The model under review builds one solid part; all positions refer to its coordinate system, in mm. Face numbers are marked on the shaded views. A direction names the side the tool comes from. Round coordinates to 2 decimals unless told otherwise and drop trailing zeros. Loops run counter-clockwise (first coordinate to the right, second up) from the corner with the lowest first, then second, coordinate; pieces in that order, holes last. Notation, with made-up numbers: (64.25, -17) -> (103.25, -17) arc R27 cw to (103.25, 0) -> close; hole circle Ø10 at (0.5, 63). An arc over 180 degrees is marked (long way). Use a Markdown table: item, result. Add a question column.
1) Mouldability with a two-part tool opening along Y and no side actions: class the marked faces 1, 2, 3 and 4 as released by +Y, released by -Y, zero draft, split by the parting line, or undercut.
2) Wall thickness on probe 1 along Y at (x, z) = (38.5, 15.5); probe 2 along X at (y, z) = (134.5, 10); probe 3 along Y at (x, z) = (46.5, 10.75): over which ranges is each line inside the solid? List them lowest first.
3) Insertion check: pin 1 (2.5 mm diameter, centred on x = 51.5, y = 134, fed in from +Z); pin 2 (2.5 mm diameter, centred on x = 51, y = 74, fed in from +Z); pin 3 (3 mm diameter, centred on y = 99.5, z = 8.5, fed in from -X). Each pin has a flat end and moves straight along its axis. Give the tip position at first contact, or say it passes through.
4) Consider section D-D on y = 122.5. Give the boundary of the cut face in (x, z).
5) For the marked faces 5, 6 and 7, list the 3-axis set-ups (+Z, -Z, +X, -X, +Y, -Y) from which the entire face can be reached by the end or side of a thin tool; tool diameter is ignored.
6) Consider section B-B on z = 1.5. State how many separate pieces and enclosed holes the cut face has, plus the area to 3 significant figures.
7) Consider section A-A on z = 8. Give the boundary of the cut face in (x, y) (3 decimals), plus the area to 3 significant figures.
8) Consider section C-C on x = 70. Give the boundary of the cut face in (y, z).
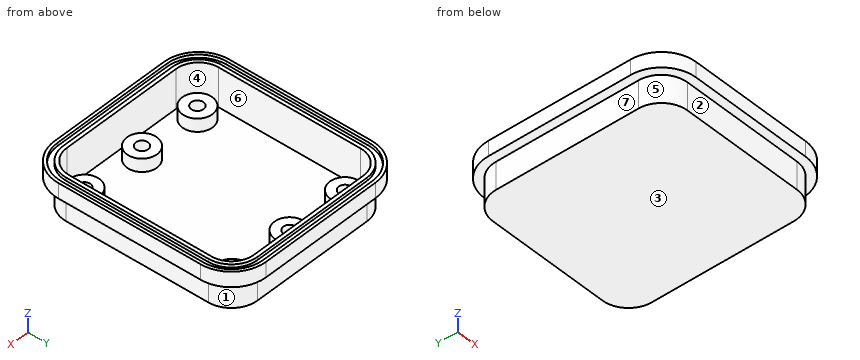
from build123d import *

# Parameters (mm, degrees)
BOSS_EXTRUDE1_DEPTH  = 16.51
SHELL1_T             = 1.524
SKETCH2_R            = 6.35
SKETCH2_R_2          = 2.608000118
BOSS_EXTRUDE2_DEPTH  = 5.5
BOSS_EXTRUDE9_DEPTH  = 1.3208
BOSS_EXTRUDE10_START = 5.08
BOSS_EXTRUDE10_DEPTH = 5.08


with BuildPart() as part:
    # Sketch1 → Boss-Extrude1 (new body)
    with BuildSketch(Plane.XY):
        with BuildLine():
            Line((26.034999985, 143.509994751), (78.104997498, 143.509994751))
            ThreePointArc((78.104997498, 143.509994751), (84.840189588, 140.720186842), (87.629997498, 133.984994751))
            Line((87.629997498, 133.984994751), (87.629997498, 73.787000793))
            ThreePointArc((87.629997498, 73.787000793), (84.840189588, 67.051808703), (78.104997498, 64.262000793))
            Line((78.104997498, 64.262000793), (26.034999985, 64.262000793))
            ThreePointArc((26.034999985, 64.262000793), (19.299807894, 67.051808703), (16.509999985, 73.787000793))
            Line((16.509999985, 73.787000793), (16.509999985, 133.984994751))
            ThreePointArc((16.509999985, 133.984994751), (19.299807894, 140.720186842), (26.034999985, 143.509994751))
        make_face()
    extrude(amount=BOSS_EXTRUDE1_DEPTH)

    # Shell1
    shell1_openings = [part.faces().sort_by_distance(p)[0] for p in [
        (52.069998741, 103.885997772, 16.51),
    ]]
    offset(amount=SHELL1_T, openings=shell1_openings, kind=Kind.INTERSECTION)

    # Sketch2 → Boss-Extrude2 (add)
    # profile 1 of 6: a face of its own
    with BuildSketch(Plane.XY):
        with Locations(Location((25.292, 135.128, 0), (0, 0, 180))):
            Circle(SKETCH2_R)
        with Locations((25.292, 135.128)):
            Circle(SKETCH2_R_2, mode=Mode.SUBTRACT)
    # profile 2 of 6: a face of its own
    with BuildSketch(Plane.XY):
        with Locations(Location((51.708, 135.128, 0), (0, 0, 180))):
            Circle(SKETCH2_R)
        with Locations((51.708, 135.128)):
            Circle(SKETCH2_R_2, mode=Mode.SUBTRACT)
    # profile 3 of 6: a face of its own
    with BuildSketch(Plane.XY):
        with Locations(Location((79.14, 135.128, 0), (0, 0, 180))):
            Circle(SKETCH2_R)
        with Locations((79.14, 135.128)):
            Circle(SKETCH2_R_2, mode=Mode.SUBTRACT)
    # profile 4 of 6: a face of its own
    with BuildSketch(Plane.XY):
        with Locations(Location((25.292, 72.644, 0), (0, 0, 180))):
            Circle(SKETCH2_R)
        with Locations((25.292, 72.644)):
            Circle(SKETCH2_R_2, mode=Mode.SUBTRACT)
    # profile 5 of 6: a face of its own
    with BuildSketch(Plane.XY):
        with Locations(Location((51.708, 72.644, 0), (0, 0, 180))):
            Circle(SKETCH2_R)
        with Locations((51.708, 72.644)):
            Circle(SKETCH2_R_2, mode=Mode.SUBTRACT)
    # profile 6 of 6: a face of its own
    with BuildSketch(Plane.XY):
        with Locations(Location((79.14, 72.644, 0), (0, 0, 180))):
            Circle(SKETCH2_R)
        with Locations((79.14, 72.644)):
            Circle(SKETCH2_R_2, mode=Mode.SUBTRACT)
    extrude(amount=BOSS_EXTRUDE2_DEPTH)



with BuildPart() as body_2:
    # Sketch7 → Boss-Extrude9 (new body)
    with BuildSketch(Plane.XY.offset(16.51)):
        with BuildLine():
            Line((92.786197498, 73.787000793), (92.786197498, 133.984994751))
            ThreePointArc((92.786197498, 133.984994751), (88.486173574, 144.366170827), (78.104997498, 148.666194751))
            Line((78.104997498, 148.666194751), (26.034999985, 148.666194751))
            ThreePointArc((26.034999985, 148.666194751), (15.653823909, 144.366170827), (11.353799985, 133.984994751))
            Line((11.353799985, 133.984994751), (11.353799985, 73.787000793))
            ThreePointArc((11.353799985, 73.787000793), (15.653823909, 63.405824718), (26.034999985, 59.105800793))
            Line((26.034999985, 59.105800793), (78.104997498, 59.105800793))
            ThreePointArc((78.104997498, 59.105800793), (88.486173574, 63.405824718), (92.786197498, 73.787000793))
        make_face()
        with BuildLine():
            ThreePointArc((26.034999985, 147.396194751), (16.551849521, 143.468145215), (12.623799985, 133.984994751))
            Line((12.623799985, 133.984994751), (12.623799985, 73.787000793))
            ThreePointArc((12.623799985, 73.787000793), (16.551849521, 64.30385033), (26.034999985, 60.375800793))
            Line((26.034999985, 60.375800793), (78.104997498, 60.375800793))
            ThreePointArc((78.104997498, 60.375800793), (87.588147961, 64.30385033), (91.516197498, 73.787000793))
            Line((91.516197498, 73.787000793), (91.516197498, 133.984994751))
            ThreePointArc((91.516197498, 133.984994751), (87.588147961, 143.468145215), (78.104997498, 147.396194751))
            Line((78.104997498, 147.396194751), (26.034999985, 147.396194751))
        make_face(mode=Mode.SUBTRACT)
    extrude(amount=-BOSS_EXTRUDE9_DEPTH)


with BuildPart() as part_1:
    add(part.part)

    add(body_2.part)  # Boss-Extrude10 merges body 2
    # Sketch8 → Boss-Extrude10 (add)
    # profile 1 of 2: a face of its own
    with BuildSketch(Plane(origin=(0, 0, 15.1892), x_dir=(-1, 0, 0), z_dir=(0, 0, -1)).offset(BOSS_EXTRUDE10_START)):
        with BuildLine():
            ThreePointArc((-78.104997498, 148.666194751), (-88.486173574, 144.366170827), (-92.786197498, 133.984994751))
            Line((-92.786197498, 133.984994751), (-92.786197498, 73.787000793))
            ThreePointArc((-92.786197498, 73.787000793), (-88.486173574, 63.405824718), (-78.104997498, 59.105800793))
            Line((-78.104997498, 59.105800793), (-26.034999985, 59.105800793))
            ThreePointArc((-26.034999985, 59.105800793), (-15.653823909, 63.405824718), (-11.353799985, 73.787000793))
            Line((-11.353799985, 73.787000793), (-11.353799985, 133.984994751))
            ThreePointArc((-11.353799985, 133.984994751), (-15.653823909, 144.366170827), (-26.034999985, 148.666194751))
            Line((-26.034999985, 148.666194751), (-78.104997498, 148.666194751))
        make_face()
        with BuildLine():
            Line((-78.104997498, 147.396194751), (-26.034999985, 147.396194751))
            ThreePointArc((-26.034999985, 147.396194751), (-16.551849521, 143.468145215), (-12.623799985, 133.984994751))
            Line((-12.623799985, 133.984994751), (-12.623799985, 73.787000793))
            ThreePointArc((-12.623799985, 73.787000793), (-16.551849521, 64.30385033), (-26.034999985, 60.375800793))
            Line((-26.034999985, 60.375800793), (-78.104997498, 60.375800793))
            ThreePointArc((-78.104997498, 60.375800793), (-87.588147961, 64.30385033), (-91.516197498, 73.787000793))
            Line((-91.516197498, 73.787000793), (-91.516197498, 133.984994751))
            ThreePointArc((-91.516197498, 133.984994751), (-87.588147961, 143.468145215), (-78.104997498, 147.396194751))
        make_face(mode=Mode.SUBTRACT)
    # profile 2 of 2: a face of its own
    with BuildSketch(Plane(origin=(0, 0, 15.1892), x_dir=(-1, 0, 0), z_dir=(0, 0, -1)).offset(BOSS_EXTRUDE10_START)):
        with BuildLine():
            ThreePointArc((-26.034999985, 147.396194751), (-16.551849521, 143.468145215), (-12.623799985, 133.984994751))
            Line((-12.623799985, 133.984994751), (-12.623799985, 73.787000793))
            ThreePointArc((-12.623799985, 73.787000793), (-16.551849521, 64.30385033), (-26.034999985, 60.375800793))
            Line((-26.034999985, 60.375800793), (-78.104997498, 60.375800793))
            ThreePointArc((-78.104997498, 60.375800793), (-87.588147961, 64.30385033), (-91.516197498, 73.787000793))
            Line((-91.516197498, 73.787000793), (-91.516197498, 133.984994751))
            ThreePointArc((-91.516197498, 133.984994751), (-87.588147961, 143.468145215), (-78.104997498, 147.396194751))
            Line((-78.104997498, 147.396194751), (-26.034999985, 147.396194751))
        make_face()
        with BuildLine():
            ThreePointArc((-26.034999985, 62.738000793), (-18.222177159, 65.974177968), (-14.985999985, 73.787000793))
            Line((-14.985999985, 73.787000793), (-14.985999985, 133.984994751))
            ThreePointArc((-14.985999985, 133.984994751), (-18.222177159, 141.797817576), (-26.034999985, 145.033994751))
            Line((-26.034999985, 145.033994751), (-78.104997498, 145.033994751))
            ThreePointArc((-78.104997498, 145.033994751), (-85.917820323, 141.797817576), (-89.153997498, 133.984994751))
            Line((-89.153997498, 133.984994751), (-89.153997498, 73.787000793))
            ThreePointArc((-89.153997498, 73.787000793), (-85.917820323, 65.974177968), (-78.104997498, 62.738000793))
            Line((-78.104997498, 62.738000793), (-26.034999985, 62.738000793))
        make_face(mode=Mode.SUBTRACT)
    extrude(amount=-BOSS_EXTRUDE10_DEPTH)


solid = part_1.part
Result set:
| question | item | result |
|---|---|---|
| 1 | face 1 | released by +Y |
| 1 | face 2 | released by -Y |
| 1 | face 3 | zero draft |
| 1 | face 4 | undercut |
| 2 | probe 1 | 59.11 to 60.38, 62.74 to 64.26, 143.51 to 145.03, 147.4 to 148.67 |
| 2 | probe 2 | 15 to 16.52, 87.62 to 89.14 |
| 2 | probe 3 | 59.11 to 64.26, 143.51 to 148.67 |
| 3 | pin 1 | z = 0 |
| 3 | pin 2 | z = 5.5 |
| 3 | pin 3 | x = 14.99 |
| 4 | outline | (11.35, 10.11) -> (14.99, 10.11) -> (14.99, -1.52) -> (89.15, -1.52) -> (89.15, 10.11) -> (92.79, 10.11) -> (92.79, 16.51) -> (91.52, 16.51) -> (91.52, 15.19) -> (89.15, 15.19) -> (89.15, 16.51) -> (87.63, 16.51) -> (87.63, 0) -> (16.51, 0) -> (16.51, 16.51) -> (14.99, 16.51) -> (14.99, 15.19) -> (12.62, 15.19) -> (12.62, 16.51) -> (11.35, 16.51) -> close |
| 5 | face 5 | -Z, -X, -Y |
| 5 | face 6 | +Z |
| 5 | face 7 | -Z, -X, +Y, -Y |
| 6 | separate pieces | 7 |
| 6 | enclosed holes | 7 |
| 6 | area | 1,070 mm2 |
| 7 | outline | (14.986, 73.787) arc R11.049 ccw to (26.035, 62.738) -> (78.105, 62.738) arc R11.049 ccw to (89.154, 73.787) -> (89.154, 133.985) arc R11.049 ccw to (78.105, 145.034) -> (26.035, 145.034) arc R11.049 ccw to (14.986, 133.985) -> close; hole (16.51, 73.787) arc R9.525 ccw to (26.035, 64.262) -> (78.105, 64.262) arc R9.525 ccw to (87.63, 73.787) -> (87.63, 133.985) arc R9.525 ccw to (78.105, 143.51) -> (26.035, 143.51) arc R9.525 ccw to (16.51, 133.985) -> close |
| 7 | area | 441 mm2 |
| 8 | outline | (59.11, 10.11) -> (62.74, 10.11) -> (62.74, -1.52) -> (145.03, -1.52) -> (145.03, 10.11) -> (148.67, 10.11) -> (148.67, 16.51) -> (147.4, 16.51) -> (147.4, 15.19) -> (145.03, 15.19) -> (145.03, 16.51) -> (143.51, 16.51) -> (143.51, 0) -> (64.26, 0) -> (64.26, 16.51) -> (62.74, 16.51) -> (62.74, 15.19) -> (60.38, 15.19) -> (60.38, 16.51) -> (59.11, 16.51) -> close |
